Geometry check sheet. Reference: the model listing, model coordinates, mm. A direction names the side the tool comes from. Give positions to 0.01 mm unless a question says otherwise; leave off trailing zeros. Order: outer loops, then holes, each group sorted by start corner. A loop starts at its lowest first (then second) coordinate and runs counter-clockwise, first axis right, second up.
```python
from build123d import *

# Parameters (mm, degrees)
SKETCH1_R            = 3.7
SKETCH1_R_2          = 2.4
PIN_SIDE_DEPTH       = 3.7
SIDE_START           = 3.7
SIDE_EAR_DEPTH       = 1
MIDDLE_RIB_DEPTH     = 0.7
SKETCH4_R            = 2.85
AXLE_BODY_DEPTH      = 3.7
AXLE_CUT_DEPTH       = 13.816785869
AXLE_CUT_DEPTH_BACK  = 13.816785869
SKETCH5_W            = 1.8
SKETCH5_H            = 1.8
AXLE_SLOT_DEPTH      = 13.816785869
AXLE_SLOT_DEPTH_BACK = 13.816785869
SKETCH7_R            = 3.1
PIN_RIM_DEPTH        = 0.8


with BuildPart() as part:
    # Sketch1 → Pin Side (new, symmetric)
    with BuildSketch(Plane.XY):
        Circle(SKETCH1_R)
        Circle(SKETCH1_R_2, mode=Mode.SUBTRACT)
    extrude(amount=PIN_SIDE_DEPTH, both=True)

    # Sketch2 → Side Ear (add)
    with BuildSketch(Plane(origin=(0, 0, 0), x_dir=(1, 0, 0), z_dir=(0, 1, 0)).offset(SIDE_START)):
        with BuildLine():
            Line((0, 3.7), (0, -3.7))
            Line((0, -3.7), (8, -3.7))
            ThreePointArc((8, -3.7), (11.7, 0), (8, 3.7))
            Line((8, 3.7), (0, 3.7))
        make_face()
    side_ear = extrude(amount=-SIDE_EAR_DEPTH)

    # Mirror1: Side Ear across plane
    add(side_ear.mirror(Plane.ZX))

    # Sketch3 → Middle Rib (add, symmetric)
    with BuildSketch(Plane.XY):
        with BuildLine():
            Line((2.529822128, -2.7), (8, -2.7))
            Line((8, -2.7), (8, 2.7))
            Line((8, 2.7), (2.529822128, 2.7))
            ThreePointArc((2.529822128, 2.7), (3.7, 0), (2.529822128, -2.7))
        make_face()
    extrude(amount=MIDDLE_RIB_DEPTH, both=True)

    # Sketch4 → Axle Body (add, symmetric)
    with BuildSketch(Plane(origin=(0, 0, 0), x_dir=(1, 0, 0), z_dir=(0, 1, 0))):
        with Locations((8, 0)):
            Circle(SKETCH4_R)
    extrude(amount=AXLE_BODY_DEPTH, both=True)

    # Sketch5 → Axle Cut (cut, two sides: drawn at the far end of the back side and taken through both)
    with BuildSketch(Plane(origin=(0, 0, 0), x_dir=(1, 0, 0), z_dir=(0, 1, 0)).offset(-AXLE_CUT_DEPTH_BACK)):
        with BuildLine():
            Line((5.775140454, -0.9), (7.1, -0.9))
            Line((7.1, -0.9), (7.1, 0.9))
            Line((7.1, 0.9), (5.775140454, 0.9))
            ThreePointArc((5.775140454, 0.9), (5.644191972, 0.458441422), (5.6, -1.6e-08))
            ThreePointArc((5.6, -1.6e-08), (5.644191976, -0.458441438), (5.775140454, -0.9))
        make_face()
        with BuildLine():
            Line((7.1, 0.9), (8.9, 0.9))
            Line((8.9, 0.9), (8.9, 2.224859546))
            ThreePointArc((8.9, 2.224859546), (8.45844143, 2.355808026), (8, 2.4))
            ThreePointArc((8, 2.4), (7.54155857, 2.355808026), (7.1, 2.224859546))
            Line((7.1, 2.224859546), (7.1, 0.9))
        make_face()
        with Locations((8, 0)):
            Rectangle(SKETCH5_W, SKETCH5_H)
        with BuildLine():
            Line((8.9, 0.9), (8.9, -0.9))
            Line((8.9, -0.9), (10.224859546, -0.9))
            ThreePointArc((10.224859546, -0.9), (10.355808026, -0.45844143), (10.4, 0))
            ThreePointArc((10.4, 0), (10.355808026, 0.45844143), (10.224859546, 0.9))
            Line((10.224859546, 0.9), (8.9, 0.9))
        make_face()
        with BuildLine():
            ThreePointArc((7.1, -2.224859546), (7.54155857, -2.355808026), (8, -2.4))
            ThreePointArc((8, -2.4), (8.45844143, -2.355808026), (8.9, -2.224859546))
            Line((8.9, -2.224859546), (8.9, -0.9))
            Line((8.9, -0.9), (7.1, -0.9))
            Line((7.1, -0.9), (7.1, -2.224859546))
        make_face()
    extrude(amount=AXLE_CUT_DEPTH + AXLE_CUT_DEPTH_BACK, mode=Mode.SUBTRACT)

    # Sketch6 → Axle Slot (cut, two sides: drawn at the far end of the back side and taken through both)
    with BuildSketch(Plane.XY.offset(-AXLE_SLOT_DEPTH_BACK)):
        with BuildLine():
            Line((7.5, -2.2), (7.5, 2.2))
            ThreePointArc((7.5, 2.2), (8, 2.7), (8.5, 2.2))
            Line((8.5, 2.2), (8.5, -2.2))
            ThreePointArc((8.5, -2.2), (8, -2.7), (7.5, -2.2))
        make_face()
    extrude(amount=AXLE_SLOT_DEPTH + AXLE_SLOT_DEPTH_BACK, mode=Mode.SUBTRACT)

    # Sketch7 → Pin Rim (cut)
    with BuildSketch(Plane.XY.offset(3.7)):
        Circle(SKETCH7_R)
    pin_rim = extrude(amount=-PIN_RIM_DEPTH, mode=Mode.SUBTRACT)

    # Mirror2: Pin Rim across plane
    add(pin_rim.mirror(Plane.XY), mode=Mode.SUBTRACT)


solid = part.part
```
Q1. Cross-section at B-B, the plane y = 0. Give the number of separate pieces and of enclosed holes in the cut face, and give its area (3 significant figures).
Q2. Release check for a two-part mould opening along X. For faces 1 (the face through (-3.7, 0.1, 0.1)), 2 (the face through (5.92, 0.04, 1.95)), 3 (the face through (11.7, 3.2, 0.1)) record: pulls with the +X half, pulls with the -X half, needs draft (parallel to the pull), parting line crosses it, or undercut.
Q3. Cross-section at C-C, the plane x = 1.25. Record the boundary of the cut face in (y, z), and give its area (3 significant figures).
Q4. Cross-section at A-A, the plane z = 3.5. Record the boundary of the cut face in (x, y).
Q5. Thickness scan on L1, parallel to Y at x = 0, z = 1; L2, parallel to Y at x = 0, z = -3.2; L3, parallel to Z at x = 7, y = -3. Record the ranges inside material, lowest first.
Q6. Access from +Z, -Z, +X, -X, +Y, -Y to the whole of each face (thin tool, end or side, straight path). Record for faces 4 (the face through (10, 0, -0.9)), 5 (the face through (4, 0, 0.7)), 6 (the face through (5, -2.7, -1)), 7 (the face through (6.271, 0.038, -2.265)).
Q7. Cross-section at D-D, the plane z = -1.25. Record the boundary of the cut face in (x, y).
Q8. Gauge pin test, flat ends, axial feed: P1, Ø0.7, axis at y = 1, z = 1.5, coming from the -X side; P2, Ø1, axis at y = -1, z = 0.5, coming from the +X side; P3, Ø0.7, axis at y = -1.5, z = -1.5, coming from the +X side. Record the tip position at first contact, or that the pin passes through.
Answers follow:
1. separate pieces: 3
1. enclosed holes: 0
1. area: 30.1 mm2
2. face 1: pulls with the -X half
2. face 2: undercut
2. face 3: pulls with the +X half
3. outline: (-3.7, -3.7) - (-2.84, -3.7) - (-2.84, -2.9) - (-2.05, -2.9) - (-2.05, 2.9) - (-2.84, 2.9) - (-2.84, 3.7) - (-3.7, 3.7) - close; (2.05, -2.9) - (2.84, -2.9) - (2.84, -3.7) - (3.7, -3.7) - (3.7, 3.7) - (2.84, 3.7) - (2.84, 2.9) - (2.05, 2.9) - close
3. area: 21.9 mm2
4. outline: (0, -3.7) - (9.2, -3.7) - (9.2, -2.7) - (2.53, -2.7) arc R3.7 ccw to (2.53, 2.7) - (9.2, 2.7) - (9.2, 3.7) - (0, 3.7) arc R3.7 ccw to start; hole circle Ø6.2 at (0, 0)
5. L1: y = -3.7 to -2.4, 2.4 to 3.7
5. L2: y = -3.7 to -3.1, 3.1 to 3.7
5. L3: z = -3.7 to -0.9, 0.9 to 3.7
6. face 4: +Y, -Y
6. face 5: +Z
6. face 6: none
6. face 7: -Z
7. outline: (0, -3.7) - (7.1, -3.7) - (7.1, 3.7) - (0, 3.7) arc R3.7 ccw to start; (8.9, -3.7) - (11.48, -3.7) - (11.48, -2.7) - (10.56, -2.7) - (10.56, 2.7) - (11.48, 2.7) - (11.48, 3.7) - (8.9, 3.7) - close; hole circle Ø4.8 at (0, 0); hole (2.53, -2.7) - (5.44, -2.7) - (5.44, 2.7) - (2.53, 2.7) arc R3.7 cw to start
8. P1: stops at x = -3.64
8. P2: stops at x = 10.85
8. P3: stops at x = 10.61
